Verification items for the finished model (mm, model axes). A direction names the side the tool comes from. Coordinates: 2 decimals unless noted, no trailing zeros. Order: outer loops, then holes, each group sorted by start corner. A loop starts at its lowest first (then second) coordinate and runs counter-clockwise, first axis right, second up. Notation, with made-up numbers: M 15,46 L 38,46 A29 cw 38,72 Z; hole C -21.5,26.25 d2. An arc over 180 degrees is marked long. Return JSON: item names as keys, results as strings.
```python
from build123d import *

# Parameters (mm, degrees)
F1_DEPTH = 3.15
F2_R     = 3.14
F5_DEPTH = 1.54
F4_R     = 1.5
F4_R_2   = 1.75
F6_DEPTH = 12.5


with BuildPart() as f1:
    # F0 (on Top) → F1 (new body, symmetric)
    with BuildSketch(Plane.XY):
        Polygon((0, 2.965), (0, 0), (0, -2.965), (-8.13, -2.965), (-8.13, -7.005), (0.41, -7.005), (0.41, -12.965), (3.13, -12.965), (3.13, 0), (3.13, 12.965), (0.41, 12.965), (0.41, 7.005), (-8.13, 7.005), (-8.13, 2.965), align=None)
    extrude(amount=F1_DEPTH, both=True)

    # F2
    f2_edges = [f1.edges().sort_by_distance(p)[0] for p in [
        (1.77, 12.965, 3.15),
        (1.77, 12.965, -3.15),
        (1.77, -12.965, 3.15),
        (1.77, -12.965, -3.15),
    ]]
    fillet(f2_edges, radius=F2_R)

    # F3 (on face) → F5 (join)
    with BuildSketch(Plane.YZ.offset(3.13)):
        with BuildLine():
            Line((-9.9, -3.67), (-9.9, -18.73))
            Line((-9.9, -18.73), (9.9, -18.73))
            Line((9.9, -18.73), (9.9, -3.67))
            ThreePointArc((9.9, -3.67), (13.57, 0), (9.9, 3.67))
            Line((9.9, 3.67), (-9.9, 3.67))
            ThreePointArc((-9.9, 3.67), (-13.57, 0), (-9.9, -3.67))
        make_face()
    extrude(amount=F5_DEPTH)

    # F4 (on face) → F6 (cut, symmetric)
    with BuildSketch(Plane.YZ.offset(3.13)):
        with Locations((-10.4, 0)):
            Circle(F4_R)
        with Locations((10.4, 0)):
            Circle(F4_R)
        with Locations((-7.75, -7.68)):
            Circle(F4_R_2)
        with Locations((7.75, -7.68)):
            Circle(F4_R_2)
    extrude(amount=F6_DEPTH, both=True, mode=Mode.SUBTRACT)


solid = f1.part
```
Q1. Material ranges on line 1 along Y through (x, z) = (3.85, 0); line 2 along Y through (x, z) = (-2.5, 1) (3 decimals); line 3 along Z through (x, y) = (-5, -6.75), recorded low to high.
Values:
{"line 1": "-13.57 to -11.9, -8.9 to 8.9, 11.9 to 13.57", "line 2": "-7.005 to -2.965, 2.965 to 7.005", "line 3": "-3.15 to 3.15"}
Q2. Cross-section at B-B, the plane z = -7.68. Record the boundary of the cut face in (x, y), and give its area (3 significant figures).
Values:
{"outline": "M 3.13,-9.9 L 4.67,-9.9 L 4.67,-9.5 L 3.13,-9.5 Z; M 3.13,-6 L 4.67,-6 L 4.67,6 L 3.13,6 Z; M 3.13,9.5 L 4.67,9.5 L 4.67,9.9 L 3.13,9.9 Z", "area": "19.7 mm^2"}
Q3. Tool access check on faces 5 (the face through (1.789, -12.07, -2.206)), 6 (the face through (1.751, 12.07, -2.206)), 7 (the face through (-4, -7.005, 0)). Record the directions out of +Z, -Z, +X, -X, +Y, -Y that give a thin tool (end or side, any length) a straight path to the whole face; none if there is none.
Values:
{"face 5": "-Z, -X, -Y", "face 6": "-Z, -X, +Y", "face 7": "+Z, -Z, -X, -Y"}
Q4. Cross-section at D-D, the plane z = 2.25. Record the boundary of the cut face in (x, y) (3 decimals), and give its area (3 significant figures).
Values:
{"outline": "M -8.13,-7.005 L 0.41,-7.005 L 0.41,-12.025 L 3.13,-12.025 L 3.13,-12.799 L 4.67,-12.799 L 4.67,12.799 L 3.13,12.799 L 3.13,12.025 L 0.41,12.025 L 0.41,7.005 L -8.13,7.005 L -8.13,2.965 L 0,2.965 L 0,-2.965 L -8.13,-2.965 Z", "area": "176 mm^2"}
Q5. Cross-section at A-A, the plane y = 7.75. Record the boundary of the cut face in (x, z).
Values:
{"outline": "M 0.41,-3.15 L 3.13,-3.15 L 3.13,-5.93 L 4.67,-5.93 L 4.67,3.67 L 3.13,3.67 L 3.13,3.15 L 0.41,3.15 Z; M 3.13,-18.73 L 4.67,-18.73 L 4.67,-9.43 L 3.13,-9.43 Z"}
Q6. Draft check along Y on faces 1 (the face through (0.41, 8.7, 0)), 2 (the face through (-4, 2.965, 0)), 3 (the face through (1.751, 12.07, 2.206)), 4 (the face through (3.89, -13.57, 0.08)). Enter one of: pulls with the +Y half, pulls with the -Y half, needs draft (parallel to the pull), parting line crosses it, or undercut.
Values:
{"face 1": "needs draft", "face 2": "undercut", "face 3": "pulls with the +Y half", "face 4": "pulls with the -Y half"}
Q7. Go/stop test with flat-tipped pins: pin 1 (6 mm diameter, centred on x = -5, z = -6.5, fed in from -Y); pin 2 (6 mm diameter, centred on x = -3.5, y = 0, fed in from -Z); pin 3 (7 mm diameter, centred on x = -4, z = -0.5, fed in from -Y) (3 decimals); pin 4 (2 mm diameter, centred on x = -3, y = 7.5, fed in from +Z). Record where each tip stops, or that it passes through.
Values:
{"pin 1": "through", "pin 2": "z = -3.15", "pin 3": "y = -7.005", "pin 4": "z = 3.15"}
Q8. Cross-section at C-C, the plane x = -1.5. Record the boundary of the cut face in (y, z) (3 decimals), and give its area (3 significant figures).
Values:
{"outline": "M -7.005,-3.15 L -2.965,-3.15 L -2.965,3.15 L -7.005,3.15 Z; M 2.965,-3.15 L 7.005,-3.15 L 7.005,3.15 L 2.965,3.15 Z", "area": "50.9 mm^2"}
